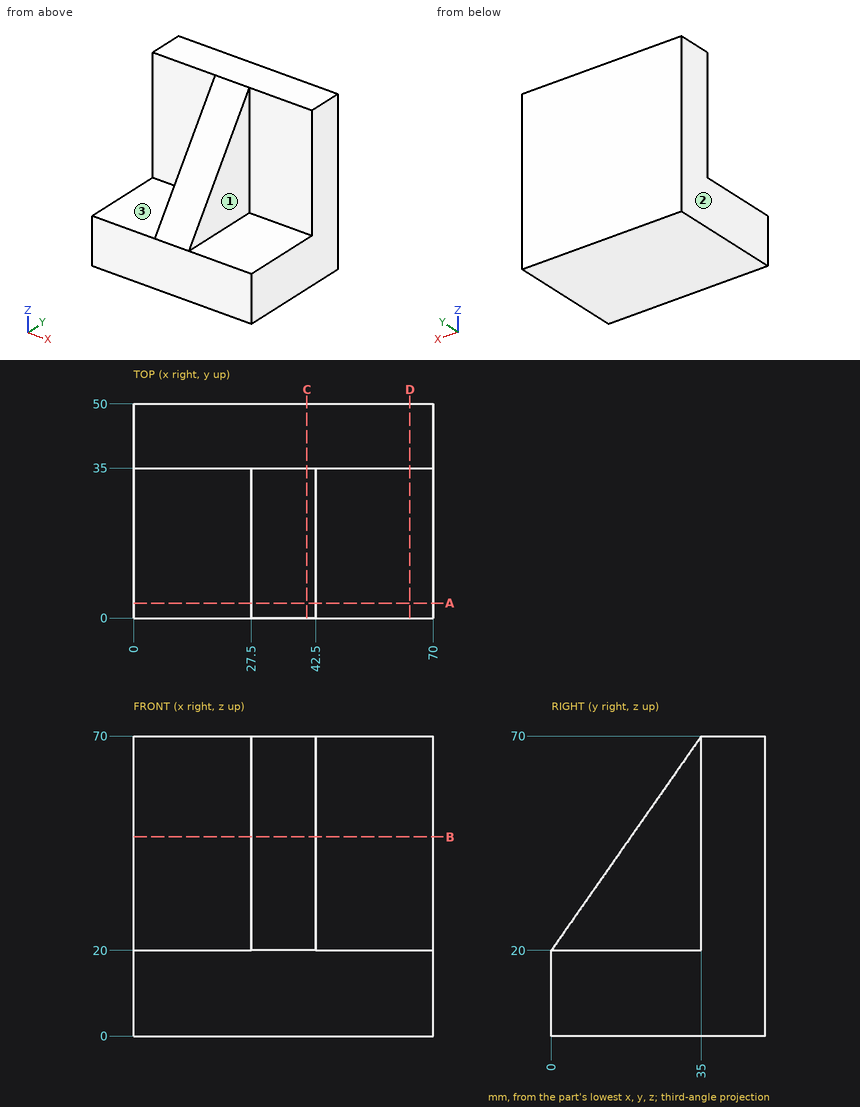
Geometry: see drawing. Coordinates: mm, zero at the bounding-box minimum. A direction names the side the tool comes from. Give positions to 0.01 mm unless a question says otherwise; leave off trailing zeros. Order: outer loops, then holes, each group sorted by start corner. A loop starts at its lowest first (then second) coordinate and runs counter-clockwise, first axis right, second up.
Q1. Section C-C on x = 40.5. Output: boundary loops of the cut face in (y, z).
Checked values:
outline: (0, 0) - (50, 0) - (50, 70) - (35, 70) - (0, 20) - close
Q2. Set-up query: the marked faces 1, 2 and 3. Return all of +Z, -Z, +X, -X, +Y, -Y with unobstructed straight access to the full face (end or side cutting, diameter ignored); none if empty.
Checked values:
face 1: +Z, +X, -Y
face 2: +Z, -Z, -X, +Y, -Y
face 3: +Z, -X, -Y
Q3. Section A-A on y = 3.5. Output: boundary loops of the cut face in (x, z), and give its area (4 significant figures).
Checked values:
outline: (0, 0) - (70, 0) - (70, 20) - (42.5, 20) - (42.5, 25) - (27.5, 25) - (27.5, 20) - (0, 20) - close
area: 1,475 mm2
Q4. Contact query for flat-ended pins moving along their axis: pin 1 Ø4 at (x, z) = (40.5, 57.5) entering from -Y; pin 2 Ø10.5 at (y, z) = (21, 52.5) entering from -X; pin 3 Ø1 at (x, z) = (39, 45.5) entering from -Y. Output: stop coordinate, or through.
Checked values:
pin 1: stops at y = 24.85
pin 2: stops at x = 27.5
pin 3: stops at y = 17.5
Q5. Section B-B on z = 46.5. Output: boundary loops of the cut face in (x, y), and give its area (3 significant figures).
Checked values:
outline: (0, 35) - (27.5, 35) - (27.5, 18.55) - (42.5, 18.55) - (42.5, 35) - (70, 35) - (70, 50) - (0, 50) - close
area: 1,300 mm2
Q6. Ray query, probe 1 along Y at (x, z) = (52, 57.5); probe 2 along Z at (x, y) = (23.5, 34.5); probe 3 along Z at (x, y) = (34.5, 21). Return the intervals inside material, ascending.
Checked values:
probe 1: y = 35 to 50
probe 2: z = 0 to 20
probe 3: z = 0 to 50
Q7. Section D-D on x = 64.5. Output: boundary loops of the cut face in (y, z).
Checked values:
outline: (0, 0) - (50, 0) - (50, 70) - (35, 70) - (35, 20) - (0, 20) - close
